For this review, take the finished solid that the model builds, in its own axes (mm). A direction names the side the tool comes from. Round coordinates to 2 decimals unless told otherwise and drop trailing zeros. Write each loop counter-clockwise with the first axis right and the second up, starting at its lowest first coordinate (ties: lowest second). Pieces come first, ordered by that corner, then holes. Notation, with made-up numbers: M 51.25,51 L 104.25,51 A35 ccw 104.25,83 Z; hole C 55.25,-23.5 d10. An arc over 180 degrees is marked long. Answer in a Markdown table with one row per item.
```python
from build123d import *

# Parameters (mm, degrees)
F0_W     = 3.2269247949
F0_H     = 3.3961120509
F0_W_2   = 3.7572830241
F0_H_2   = 3.6561227749
F0_W_3   = 4.8879086971
F0_H_3   = 7.111184299
F0_W_4   = 1.7087571323
F0_H_4   = 4.5836493373
F0_W_5   = 16.8966799974
F0_H_5   = 15.7367065549
F0_W_6   = 1.7694719136
F0_H_6   = 1.0562464595
F0_W_7   = 1.1583864689
F0_H_7   = 0.9117685258
F0_W_8   = 1.178054139
F0_H_8   = 2.6293583214
F1_DEPTH = 25.4


with BuildPart() as f1:
    # F0 (on Front) → F1 (new body)
    with BuildSketch(Plane.XZ):
        Polygon((37.3980215415, -20.2466417104), (37.3980215415, 27.6115918206), (-37.3980215415, 27.6115918206), (-37.3980215415, 23.2865139842), (-37.3980215415, -16.2047892809), (-37.3980215415, -27.6115918206), (-28.3106606554, -27.6115918206), (21.8509719518, -27.6115918206), (30.9441719518, -27.6115918206), (37.3980215415, -27.6115918206), align=None)
        Polygon((37.3980215415, 32.7450931072), (37.3980215415, 27.6115918206), (37.3980215415, -20.2466417104), (42.4228385091, -20.2466417104), (42.4228385091, -10.5181215331), (42.4228385091, 32.7450931072), align=None)
        Polygon((-37.3980215415, -16.2047892809), (-37.3980215415, 23.2865139842), (-41.2078462541, 23.2865139842), (-41.2078462541, 15.1224471629), (-41.2078462541, -16.2047892809), align=None)
        Polygon((42.4228385091, 37.7946980298), (42.4228385091, 32.7450931072), (42.4228385091, -10.5181215331), (47.24393785, -10.5181215331), (47.24393785, 3.5339901224), (47.24393785, 37.7946980298), align=None)
        Polygon((30.9441719518, -35.5871918206), (30.9441719518, -27.6115918206), (21.8509719518, -27.6115918206), (21.8509719518, -35.5871918206), (21.8509719518, -43.5627918206), (30.9441719518, -43.5627918206), align=None)
        Polygon((-28.3106606554, -27.6115918206), (-37.3980215415, -27.6115918206), (-37.3980215415, -44.3883202384), (-28.3106606554, -44.3883202384), (-28.3106606554, -35.9999560295), align=None)
        Polygon((-41.2078462541, -21.7107832432), (-41.2078462541, -16.2047892809), (-41.2078462541, 15.1224471629), (-45.0683757663, 15.1224471629), (-45.0683757663, 7.9709775746), (-45.0683757663, -21.7107832432), align=None)
        Polygon((37.3980215415, -35.5871918206), (30.9441719518, -35.5871918206), (30.9441719518, -43.5627918206), (34.1710967466, -43.5627918206), (34.1710967466, -40.1666797698), (37.3980215415, -40.1666797698), align=None)
        Polygon((47.24393785, 44.3825013936), (47.24393785, 37.7946980298), (47.24393785, 3.5339901224), (52.0987957716, 3.5339901224), (52.0987957716, 20.2638655901), (52.0987957716, 44.3825013936), align=None)
        Polygon((-20.7960946072, -35.9999560295), (-28.3106606554, -35.9999560295), (-28.3106606554, -44.3883202384), (-24.5533776313, -44.3883202384), (-24.5533776313, -40.7321974635), (-20.7960946072, -40.7321974635), align=None)
        Polygon((-45.0683757663, -26.9003435969), (-45.0683757663, -21.7107832432), (-45.0683757663, 7.9709775746), (-49.1187684238, 7.9709775746), (-49.1187684238, -6.9015473127), (-49.1187684238, -26.9003435969), align=None)
        with Locations((35.7845591441, -41.8647357952)):
            Rectangle(F0_W, F0_H)
        Polygon((52.0987957716, 51.3773448765), (52.0987957716, 44.3825013936), (52.0987957716, 20.2638655901), (57.0190772414, 20.2638655901), (57.0190772414, 28.7094209343), (57.0190772414, 35.8206052333), (57.0190772414, 51.3773448765), align=None)
        with Locations((-22.6747361192, -42.5602588509)):
            Rectangle(F0_W_2, F0_H_2)
        Polygon((-49.1187684238, -34.8745509982), (-49.1187684238, -26.9003435969), (-49.1187684238, -6.9015473127), (-52.5362826884, -6.9015473127), (-52.5362826884, -24.2168344557), (-52.5362826884, -34.8745509982), (-50.8275255561, -34.8745509982), align=None)
        Polygon((57.0190772414, 61.949711293), (57.0190772414, 51.3773448765), (57.0190772414, 35.8206052333), (61.9069859385, 35.8206052333), (61.9069859385, 40.3074584901), (61.9069859385, 61.949711293), align=None)
        with Locations((59.46303159, 32.2650130838)):
            Rectangle(F0_W_3, F0_H_3)
        with Locations((-51.6819041222, -37.1663756669)):
            Rectangle(F0_W_4, F0_H_4)
        Polygon((-52.5362826884, -34.8745509982), (-52.5362826884, -24.2168344557), (-55.3043186665, -24.2168344557), (-55.3043186665, -32.844690606), (-55.3043186665, -39.8848950863), (-55.3043186665, -40.9411415458), (-55.3043186665, -41.4725467563), (-52.5362826884, -41.4725467563), (-52.5362826884, -39.4582003355), align=None)
        Polygon((61.9069859385, 73.9622488618), (61.9069859385, 61.949711293), (61.9069859385, 40.3074584901), (66.6303560138, 40.3074584901), (66.6303560138, 58.2255423069), (66.6303560138, 73.9622488618), align=None)
        Polygon((-55.3043186665, -39.8848950863), (-55.3043186665, -32.844690606), (-57.7685758471, -32.844690606), (-57.7685758471, -38.2937081158), (-57.7685758471, -39.2054766417), (-57.7685758471, -39.8848950863), (-57.07379058, -39.8848950863), align=None)
        with Locations((75.0786960125, 66.0938955843)):
            Rectangle(F0_W_5, F0_H_5)
        with Locations((-56.1890546232, -40.413018316)):
            Rectangle(F0_W_6, F0_H_6)
        Polygon((-57.7685758471, -38.2937081158), (-57.7685758471, -32.844690606), (-57.7685758471, -29.8693664372), (-60.0853487849, -29.8693664372), (-60.0853487849, -34.0815372765), (-60.0853487849, -36.7108955979), (-60.0853487849, -38.2937081158), (-58.926962316, -38.2937081158), align=None)
        with Locations((-58.3477690816, -38.7495923787)):
            Rectangle(F0_W_7, F0_H_7)
        Polygon((-60.0853487849, -34.0815372765), (-60.0853487849, -29.8693664372), (-60.0853487849, -26.6751870513), (-62.441457063, -26.6751870513), (-62.441457063, -34.0815372765), (-61.2634029239, -34.0815372765), align=None)
        with Locations((-60.6743758544, -35.3962164372)):
            Rectangle(F0_W_8, F0_H_8)
    extrude(amount=F1_DEPTH)


solid = f1.part
```
Q1. Take a section at B-B (x = 29). State the section outline as (y, z) points, then the cut area to 3 significant figures.
Found:
| item | result |
|---|---|
| outline | M -25.4,-43.56 L 0,-43.56 L 0,27.61 L -25.4,27.61 Z |
| area | 1,810 mm² |
Q2. For probe 1 along Z at (x, y) = (-23.5, -21.25); probe 2 along X at (y, z) = (-16.25, -24.5); probe 3 along Z at (x, y) = (35, -22.25), list the stretches that pass through material, from the lowest coordinate up.
Found:
| item | result |
|---|---|
| probe 1 | -44.39 to -36, -27.61 to 27.61 |
| probe 2 | -55.3 to -45.07, -37.4 to 37.4 |
| probe 3 | -43.56 to -35.59, -27.61 to 27.61 |
Q3. Machinability: for faces 5 (the face through (34, -13, -27.612)), 6 (the face through (-49.119, -13, 1)), 7 (the face through (52.099, -13, 12)), which of the approach directions +Z, -Z, +X, -X, +Y, -Y give a long, thin tool a straight path to every point of the face, cutting with its end or side? Answer none if there is none.
Found:
| item | result |
|---|---|
| face 5 | +X, +Y, -Y |
| face 6 | +Z, -X, +Y, -Y |
| face 7 | -Z, +X, +Y, -Y |
Q4. Insertion check: P1, Ø5.5, axis at y = -7.5, z = 35, coming from the -X side; P2, Ø5, axis at x = 53, y = -6.5, coming from the +Z side; P3, Ø2.5, axis at x = 55.5, y = -18.5, coming from the -Z side; P4, Ø5, axis at x = -39, z = -9.5, coming from the +Y side. Each pin has a flat end and moves straight along its axis. Give the tip position at first contact, or say it passes through.
Found:
| item | result |
|---|---|
| P1 | x = 37.4 |
| P2 | z = 51.38 |
| P3 | z = 20.26 |
| P4 | y = 0 |
Q5. Mouldability with a two-part tool opening along X and no side actions: class faces 1 (the face through (-37.398, -13, -30)), 2 (the face through (1, -13, 27.612)), 3 (the face through (52.099, -13, 48)), 4 (the face through (-49.119, -13, -31)) as +X half, -X half, draft (parallel to the pull), parting line (faces both ways), or undercut.
Found:
| item | result |
|---|---|
| face 1 | undercut |
| face 2 | draft |
| face 3 | -X half |
| face 4 | undercut |
Q6. Take a section at A-A (z = 17). State the section outline as (x, y) points.
Found:
| item | result |
|---|---|
| outline | M -41.21,-25.4 L 52.1,-25.4 L 52.1,0 L -41.21,0 Z |
